CAD build for the part. Positions are in the model's coordinates, mm. Round coordinates to 2 decimals unless told otherwise and drop trailing zeros. Order: outer loops, then holes, each group sorted by start corner. A loop starts at its lowest first (then second) coordinate and runs counter-clockwise, first axis right, second up. Notation, with made-up numbers: (42, -34.75) - (60, -34.75) arc R18 ccw to (60, -28.75) - close; hole circle Ø1 at (16, 1.25). An arc over 180 degrees is marked (long way). Write item = value, one per line.
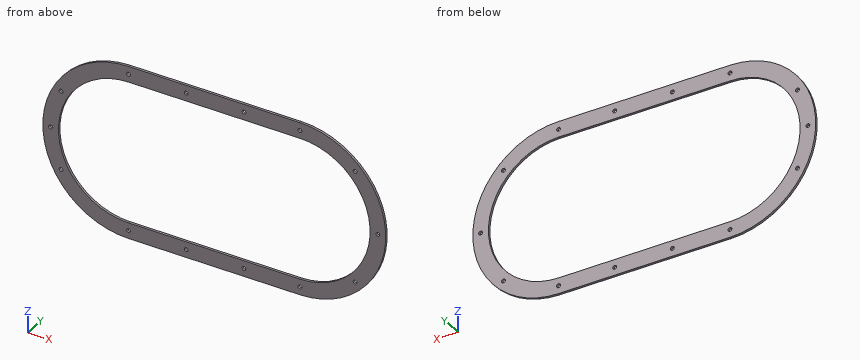
from build123d import *

# Parameters (mm, degrees)
ESBO_O1_R                = 2.5
RESSALTO_EXTRUS_O2_DEPTH = 3


with BuildPart() as part:
    # Esboço1 → Ressalto-extrusão2 (new body)
    with BuildSketch(Plane(origin=(0, 0, 0), x_dir=(1, 0, 0), z_dir=(0, 1, 0))):
        with BuildLine():
            Line((68.54446848, 235.010465991), (288.54446848, 235.010465991))
            ThreePointArc((288.54446848, 235.010465991), (398.54446848, 125.010465991), (288.54446848, 15.010465991))
            Line((288.54446848, 15.010465991), (68.54446848, 15.010465991))
            ThreePointArc((68.54446848, 15.010465991), (-41.45553152, 125.010465991), (68.54446848, 235.010465991))
        make_face()
        with Locations(Location((68.54446848, 225.010465991, 0), (0, 0, 270))):
            Circle(ESBO_O1_R, mode=Mode.SUBTRACT)
        with Locations(Location((68.54446848, 25.010465991, 0), (0, 0, 270))):
            Circle(ESBO_O1_R, mode=Mode.SUBTRACT)
        with Locations(Location((288.54446848, 25.010465991, 0), (0, 0, 270))):
            Circle(ESBO_O1_R, mode=Mode.SUBTRACT)
        with Locations(Location((288.54446848, 225.010465991, 0), (0, 0, 270))):
            Circle(ESBO_O1_R, mode=Mode.SUBTRACT)
        with Locations(Location((-18.058071899, 175.010465991, 0), (0, 0, 270))):
            Circle(ESBO_O1_R, mode=Mode.SUBTRACT)
        with Locations(Location((-31.45553152, 125.010465991, 0), (0, 0, 270))):
            Circle(ESBO_O1_R, mode=Mode.SUBTRACT)
        with Locations(Location((-18.058071899, 75.010465991, 0), (0, 0, 270))):
            Circle(ESBO_O1_R, mode=Mode.SUBTRACT)
        with Locations(Location((359.255146599, 54.299787872, 0), (0, 0, 270))):
            Circle(ESBO_O1_R, mode=Mode.SUBTRACT)
        with Locations(Location((388.54446848, 125.010465991, 0), (0, 0, 270))):
            Circle(ESBO_O1_R, mode=Mode.SUBTRACT)
        with Locations(Location((359.255146599, 195.72114411, 0), (0, 0, 270))):
            Circle(ESBO_O1_R, mode=Mode.SUBTRACT)
        with Locations(Location((142.54446848, 25.010465991, 0), (0, 0, 270))):
            Circle(ESBO_O1_R, mode=Mode.SUBTRACT)
        with Locations(Location((216.54446848, 25.010465991, 0), (0, 0, 270))):
            Circle(ESBO_O1_R, mode=Mode.SUBTRACT)
        with Locations(Location((142.54446848, 225.010465991, 0), (0, 0, 270))):
            Circle(ESBO_O1_R, mode=Mode.SUBTRACT)
        with Locations(Location((216.54446848, 225.010465991, 0), (0, 0, 270))):
            Circle(ESBO_O1_R, mode=Mode.SUBTRACT)
        with BuildLine():
            Line((68.54446848, 215.010465991), (288.54446848, 215.010465991))
            ThreePointArc((288.54446848, 215.010465991), (378.54446848, 125.010465991), (288.54446848, 35.010465991))
            Line((288.54446848, 35.010465991), (68.54446848, 35.010465991))
            ThreePointArc((68.54446848, 35.010465991), (-21.45553152, 125.010465991), (68.54446848, 215.010465991))
        make_face(mode=Mode.SUBTRACT)
    extrude(amount=RESSALTO_EXTRUS_O2_DEPTH)


solid = part.part
(1) Band-saw the part on B-B on z = -153.5. List the corners of the cut face in (x, y).
Solved:
outline = (-37.7, 0) - (-16.83, 0) - (-16.83, 3) - (-37.7, 3) - close; (373.92, 0) - (394.79, 0) - (394.79, 3) - (373.92, 3) - close
(2) Probe line 1 along Z through (x, y) = (68, 2.6); line 2 along Z through (x, y) = (136, 0.6); line 3 along X through (y, z) = (0.75, -23.5). List the from-to ranges inside material, lowest first.
Solved:
line_1 = -235.01 to -227.45, -222.57 to -215.01, -35.01 to -27.45, -22.57 to -15.01
line_2 = -235.01 to -215.01, -35.01 to -15.01
line_3 = 26.17 to 66.55, 70.54 to 140.55, 144.54 to 214.55, 218.54 to 286.55, 290.54 to 330.92
(3) Band-saw the part on A-A on x = 129.5. List the corners of the cut face in (y, z).
Solved:
outline = (0, -235.01) - (3, -235.01) - (3, -215.01) - (0, -215.01) - close; (0, -35.01) - (3, -35.01) - (3, -15.01) - (0, -15.01) - close
(4) Drop flat-ended pins along their axis: pin 1 (4.5 mm diameter, centred on x = 216.54, z = -225.01, fed in from -Y); pin 2 (1.5 mm diameter, centred on y = 2, z = -175.5, fed in from -X). Give the stop position or say it passes through.
Solved:
pin_1 = through
pin_2 = -29.57
(5) Band-saw the part on C-C on y = 0.75. Count the separate pieces of the cut face and the enclosed holes in it, plus the area to 3 significant figures.
Solved:
separate_pieces = 1
enclosed_holes = 15
area = 21,100 mm²
